Design review of the part built by this model. Coordinates are the model's own, in mm. A direction names the side the tool comes from. Give positions to 0.01 mm unless a question says otherwise; leave off trailing zeros. Write each loop counter-clockwise with the first axis right and the second up, starting at its lowest first coordinate (ties: lowest second). Pieces come first, ordered by that corner, then holes. Notation, with made-up numbers: (80.25, 44) -> (91.25, 44) arc R18 cw to (91.25, 72) -> close; hole circle Ø4 at (12.25, 16). An arc over 180 degrees is marked (long way). Write each question's results on one line, items separated by ' | '. Start each with the question number.
(1) Take a section at C-C (y = 17.5). State the section outline as (x, z) points.
(2) Mouldability with a two-part tool opening along X and no side actions: class faces 4 (the face through (-1, 11, -4.762)), 5 (the face through (39.514, -7.323, -6.328)), 6 (the face through (-22.54, 20.59, -6.33)) as released by +X, released by -X, zero draft, split by the parting line, or undercut.
(3) Clearance check with flat-ended pins moving along their axes: pin 1 (1.5 mm diameter, centred on x = 15, z = -5.5, fed in from +Y); pin 2 (1.5 mm diameter, centred on y = 7, z = -7, fed in from -X); pin 3 (2.5 mm diameter, centred on x = 0, y = 42.545, fed in from +Z); pin 4 (1 mm diameter, centred on y = 22, z = -6, fed in from +X). State where each tip first meets the part, or that it passes through.
(4) Take a section at B-B (z = -5.75). State the section outline as (x, y) points (1 decimal).
(5) Take a section at D-D (y = -7.8). State the section outline as (x, z) points.
(6) For faces 1 (the face through (18.26, -8.61, -6.33)), 2 (the face through (0.062, 47.307, -6.328)), 3 (the face through (-4.762, 16, -6)), list the 3-axis set-ups (+Z, -Z, +X, -X, +Y, -Y) from which the entire face can be reached by the end or side of a thin tool; tool diameter is ignored.
(7) To check wall thickness, follow probe 1 along X at (y, z) = (18.5, -5.35); probe 2 along X at (y, z) = (4, -7.2); probe 3 along Y at (x, z) = (-21, -5.2). State the ranges of each line that lie inside material, in increasing order.
(8) Take a section at A-A (x = 38). State the section outline as (y, z) points.
from build123d import *

# Parameters (mm, degrees)
BOSS_EXTRUDE2_START = -4.7625
SKETCH1_R           = 1.5875
BOSS_EXTRUDE2_DEPTH = 3.175


with BuildPart() as part:
    # Sketch1 → Boss-Extrude2 (new body)
    with BuildSketch(Plane.XY.offset(BOSS_EXTRUDE2_START)):
        with BuildLine():
            Line((-37.042399359, -12.465233892), (0, -4.861794023))
            Line((0, -4.861794023), (37.042399359, -12.465233892))
            ThreePointArc((37.042399359, -12.465233892), (42.026572193, -10.343250405), (41.801238825, -4.93085559))
            Line((41.801238825, -4.93085559), (3.801238825, 45.41414441))
            ThreePointArc((3.801238825, 45.41414441), (0, 47.3075), (-3.801238825, 45.41414441))
            Line((-3.801238825, 45.41414441), (-41.801238825, -4.93085559))
            ThreePointArc((-41.801238825, -4.93085559), (-42.026572193, -10.343250405), (-37.042399359, -12.465233892))
        make_face()
        with Locations((38, -7.8)):
            Circle(SKETCH1_R, mode=Mode.SUBTRACT)
        Circle(SKETCH1_R, mode=Mode.SUBTRACT)
        with Locations((-38, -7.8)):
            Circle(SKETCH1_R, mode=Mode.SUBTRACT)
        with Locations((0, 42.545)):
            Circle(SKETCH1_R, mode=Mode.SUBTRACT)
        Polygon((-4.7625, 3.884228234), (-4.7625, 28.330028455), (-26.596802701, -0.597549689), align=None, mode=Mode.SUBTRACT)
        Polygon((4.7625, 3.884228234), (4.7625, 28.330028455), (26.596802701, -0.597549689), align=None, mode=Mode.SUBTRACT)
    extrude(amount=-BOSS_EXTRUDE2_DEPTH)


solid = part.part
Report:
1) outline: (-24.87, -7.94) -> (-12.94, -7.94) -> (-12.94, -4.76) -> (-24.87, -4.76) -> close; (-4.76, -7.94) -> (4.76, -7.94) -> (4.76, -4.76) -> (-4.76, -4.76) -> close; (12.94, -7.94) -> (24.87, -7.94) -> (24.87, -4.76) -> (12.94, -4.76) -> close
2) face 4: zero draft | face 5: undercut | face 6: released by -X
3) pin 1: y = 31.57 | pin 2: x = -33.36 | pin 3: through | pin 4: x = 21.85
4) outline: (-41.8, -4.9) arc R4.8 ccw to (-37, -12.5) -> (0, -4.9) -> (37, -12.5) arc R4.8 ccw to (41.8, -4.9) -> (3.8, 45.4) arc R4.8 ccw to (-3.8, 45.4) -> close; hole circle Ø3.2 at (-38, -7.8); hole (-26.6, -0.6) -> (-4.8, 3.9) -> (-4.8, 28.3) -> close; hole circle Ø3.2 at (0, 0); hole circle Ø3.2 at (0, 42.5); hole (4.8, 3.9) -> (26.6, -0.6) -> (4.8, 28.3) -> close; hole circle Ø3.2 at (38, -7.8)
5) outline: (-42.76, -7.94) -> (-39.59, -7.94) -> (-39.59, -4.76) -> (-42.76, -4.76) -> close; (-36.41, -7.94) -> (-14.31, -7.94) -> (-14.31, -4.76) -> (-36.41, -4.76) -> close; (14.31, -7.94) -> (36.41, -7.94) -> (36.41, -4.76) -> (14.31, -4.76) -> close; (39.59, -7.94) -> (42.76, -7.94) -> (42.76, -4.76) -> (39.59, -4.76) -> close
6) face 1: +Z, -Z, -Y | face 2: +Z, -Z, +Y | face 3: +Z, -Z
7) probe 1: -24.12 to -12.18, -4.76 to 4.76, 12.18 to 24.12 | probe 2: -35.06 to -23.13, -4.76 to 4.76, 23.13 to 35.06 | probe 3: -9.17 to 0.55, 6.82 to 22.63
8) outline: (-12.56, -7.94) -> (-9.39, -7.94) -> (-9.39, -4.76) -> (-12.56, -4.76) -> close; (-6.21, -7.94) -> (0.11, -7.94) -> (0.11, -4.76) -> (-6.21, -4.76) -> close
